Design review of the part built by this model. Coordinates are the model's own, in mm. Round coordinates to 2 decimals unless told otherwise and drop trailing zeros. Order: outer loops, then holes, each group sorted by start corner. A loop starts at its lowest first (then second) coordinate and runs counter-clockwise, first axis right, second up. Notation, with made-up numbers: (20, -16) - (40, -16) arc R25 ccw to (40, 5) - close; hole circle Ø1 at (82.5, -39.5). An arc over 180 degrees is marked (long way). Answer as a JSON object with one key per item and string values. Group by question number.
from build123d import *

# Parameters (mm, degrees)
SKETCH1_W           = 50.8
SKETCH1_H           = 50.8
BOSS_EXTRUDE1_DEPTH = 10
SKETCH2_R           = 7
SKETCH2_R_2         = 1.5
CUT_EXTRUDE1_DEPTH  = 38.286995052
SKETCH3_R           = 1.5
CUT_EXTRUDE2_DEPTH  = 58.669749436


with BuildPart() as part:
    # Sketch1 → Boss-Extrude1 (new body)
    with BuildSketch(Plane(origin=(0, 0, 0), x_dir=(1, 0, 0), z_dir=(0, 1, 0))):
        Rectangle(SKETCH1_W, SKETCH1_H)
    extrude(amount=BOSS_EXTRUDE1_DEPTH)

    # Sketch2 → Cut-Extrude1 (cut, through all)
    with BuildSketch(Plane(origin=(0, 10, 0), x_dir=(1, 0, 0), z_dir=(0, 1, 0))):
        with Locations(Location((0, -0.172221673, 0), (0, 0, 270))):
            Circle(SKETCH2_R)
        with Locations(Location((-12.5, -0.087466912, 0), (0, 0, 270))):
            Circle(SKETCH2_R_2)
        with Locations(Location((12.5, -0.087466912, 0), (0, 0, 90))):
            Circle(SKETCH2_R_2)
    extrude(amount=-CUT_EXTRUDE1_DEPTH, mode=Mode.SUBTRACT)

    # Sketch3 → Cut-Extrude2 (cut, through all)
    with BuildSketch(Plane(origin=(0, 0, -25.4), x_dir=(-1, 0, 0), z_dir=(0, 0, -1))):
        with Locations((20, 5)):
            Circle(SKETCH3_R)
        with Locations(Location((-20, 5, 0), (0, 0, 180))):
            Circle(SKETCH3_R)
    extrude(amount=-CUT_EXTRUDE2_DEPTH, mode=Mode.SUBTRACT)


solid = part.part
1. Take a section at D-D, the plane x = 12.5. Give the boundary of the cut face in (y, z).
2. Mouldability with a two-part tool opening along X and no side actions: class faces 1 (the cylindrical face through (18.5, 4.93, -0.36)), 2 (the flat face through (25.4, 5, 0)), 3 (the flat face through (5, 10, -6)), 4 (the cylindrical face through (-2.68, 5.07, 6.64)) as pulls with the +X half, pulls with the -X half, needs draft (parallel to the pull), parting line crosses it, or undercut.
3. Take a section at A-A, the plane x = -20. Give the boundary of the cut face in (y, z), then the cut area to 3 significant figures.
4. To check wall thickness, follow line 1 (Y direction, x = -20, z = 11.5); line 2 (X direction, y = 4.25, z = -14); line 3 (Z direction, x = -4.5, y = 1.5). State the ranges of each line that lie inside material, in increasing order. Write a range as from..to.
5. Take a section at C-C, the plane z = 21.5. Give the boundary of the cut face in (x, y), then the cut area to 3 significant figures.
6. Take a section at B-B, the plane z = -6. Give the boundary of the cut face in (x, y), then the cut area to 3 significant figures.
7. Clearance check with flat-ended pins moving along their axes: P1, Ø2.5, axis at x = -12.5, z = 0.09, coming from the -Y side; P2, Ø4, axis at x = -20, y = 5, coming from the -Z side. State where each tip first meets the part, or that it passes through.
Response values:
{
 "1": {"outline": "(0, -25.4) - (10, -25.4) - (10, -1.41) - (0, -1.41) - close; (0, 1.59) - (10, 1.59) - (10, 25.4) - (0, 25.4) - close"},
 "2": {"face 1": "undercut", "face 2": "pulls with the +X half", "face 3": "needs draft", "face 4": "undercut"},
 "3": {"outline": "(0, -25.4) - (3.5, -25.4) - (3.5, 25.4) - (0, 25.4) - close; (6.5, -25.4) - (10, -25.4) - (10, 25.4) - (6.5, 25.4) - close", "area": "356 mm2"},
 "4": {"line 1": "0..3.5, 6.5..10", "line 2": "-25.4..-21.3, -18.7..18.7, 21.3..25.4", "line 3": "-25.4..-5.19, 5.53..25.4"},
 "5": {"outline": "(-25.4, 0) - (25.4, 0) - (25.4, 10) - (-25.4, 10) - close; hole circle Ø3 at (-20, 5); hole circle Ø3 at (20, 5)", "area": "494 mm2"},
 "6": {"outline": "(-25.4, 0) - (-3.3, 0) - (-3.3, 10) - (-25.4, 10) - close; (3.3, 0) - (25.4, 0) - (25.4, 10) - (3.3, 10) - close; hole circle Ø3 at (-20, 5); hole circle Ø3 at (20, 5)", "area": "428 mm2"},
 "7": {"P1": "through", "P2": "z = -25.4"}
}
